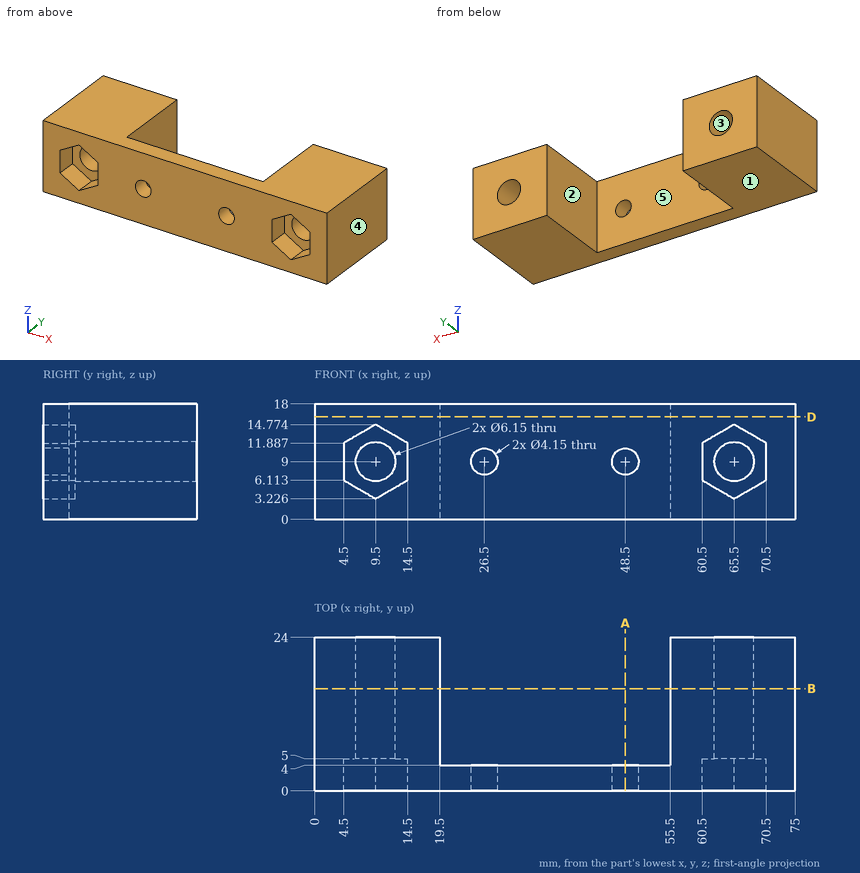
Print and shaded views of the part. All mm, measured from the part's lowest x, y and z. A direction names the side the tool comes from. Round coordinates to 2 decimals unless told otherwise and drop trailing zeros. Write each loop counter-clockwise with the first axis right and the second up, starting at its lowest first coordinate (ties: lowest second). Pieces come first, ordered by that corner, then holes. Notation, with made-up numbers: (46.5, 26) -> (57.5, 26) arc R25 cw to (57.5, 49) -> close; hole circle Ø7 at (38, 30.5). An arc over 180 degrees is marked (long way). Answer in a Markdown table with one row per item. Add a question column.
Item 1: Drill centre lines: line 1 (X direction, y = 16.75, z = 9) (1 decimal); line 2 (X direction, y = 4.5, z = 7.5); line 3 (X direction, y = 3.5, z = 11.5). Where is each one in solid material? Low to high. Write a range as from..to.
Item 2: Drop flat-ended pins along their axis: pin 1 Ø7 at (x, z) = (9.5, 9) entering from +Y; pin 2 Ø8 at (x, z) = (37.5, 12.5) entering from +Y. Give the stop position or say it passes through.
Item 3: Saw through at B-B, the plane y = 16. Count the separate pieces of the cut face and the enclosed holes in it.
Item 4: Which spindle directions (+Z, -Z, +X, -X, +Y, -Y) get a long thin tool onto all of the face, cutting with end or side? Do the marked faces 4 and 5. Say none if no direction does.
Item 5: Mould opens along Z. For the marked faces 1, 2 and 3 say: pulls with the +Z half, pulls with the -Z half, needs draft (parallel to the pull), parting line crosses it, or undercut.
Item 6: Saw through at D-D, the plane z = 16. Write the cut outline in (x, y), then the cut area to 3 significant figures.
Item 7: Saw through at A-A, the plane x = 48.5. Write the cut outline in (y, z) (1 decimal), then the cut area to 3 significant figures.
Findings below:
| question | item | result |
|---|---|---|
| 1 | line 1 | x = 0..6.4, 12.6..19.5, 55.5..62.4, 68.6..75 |
| 1 | line 2 | x = 0..4.5, 14.5..19.5, 55.5..60.5, 70.5..75 |
| 1 | line 3 | x = 0..4.5, 14.5..60.5, 70.5..75 |
| 2 | pin 1 | stops at y = 24 |
| 2 | pin 2 | stops at y = 4 |
| 3 | separate pieces | 2 |
| 3 | enclosed holes | 2 |
| 4 | face 4 | +Z, -Z, +X, +Y, -Y |
| 4 | face 5 | +Z, -Z, +Y |
| 5 | face 1 | pulls with the -Z half |
| 5 | face 2 | needs draft |
| 5 | face 3 | undercut |
| 6 | outline | (0, 0) -> (75, 0) -> (75, 24) -> (55.5, 24) -> (55.5, 4) -> (19.5, 4) -> (19.5, 24) -> (0, 24) -> close |
| 6 | area | 1,080 mm^2 |
| 7 | outline | (0, 0) -> (4, 0) -> (4, 6.9) -> (0, 6.9) -> close; (0, 11.1) -> (4, 11.1) -> (4, 18) -> (0, 18) -> close |
| 7 | area | 55.4 mm^2 |
